Source: CAD feature listing. Evaluate the final solid. Frame: model axes, mm. A direction names the side the tool comes from. Give positions to 0.01 mm unless a question says otherwise; leave off trailing zeros. Order: outer loops, then holes, each group sorted by start corner. A loop starts at its lowest first (then second) coordinate and runs counter-clockwise, first axis right, second up. Notation, with made-up numbers: (11.5, 68) - (47.5, 68) arc R33 ccw to (47.5, 97) - close; hole circle Ø7 at (7, -25). An arc over 180 degrees is marked (long way). Use CSV: the item, a comma, the result in double quotes.
```python
from build123d import *

# Parameters (mm, degrees)
ESBO_O1_R                = 1.55
RESSALTO_EXTRUS_O1_DEPTH = 6
ESBO_O2_R                = 1.6
CORTE_EXTRUS_O1_DEPTH    = 10


with BuildPart() as part:
    # Esboço1 → Ressalto-extrusão1 (new body)
    with BuildSketch(Plane.XY):
        with BuildLine():
            Line((-117, -30), (-106, -30))
            ThreePointArc((-106, -30), (-80, -5.923190379), (-54, -30))
            Line((-54, -30), (0, -30))
            Line((0, -30), (54, -30))
            ThreePointArc((54, -30), (80, -5.923190379), (106, -30))
            Line((106, -30), (117, -30))
            Line((117, -30), (117, -14.523190379))
            Line((117, -14.523190379), (113, -14.523190379))
            Line((113, -14.523190379), (113, -15.923190379))
            Line((113, -15.923190379), (110, -15.923190379))
            Line((110, -15.923190379), (110, -14.523190379))
            Line((110, -14.523190379), (106, -14.523190379))
            Line((106, -14.523190379), (106, -11.323190379))
            Line((106, -11.323190379), (110, -11.323190379))
            Line((110, -11.323190379), (110, -9.923190379))
            Line((110, -9.923190379), (113, -9.923190379))
            Line((113, -9.923190379), (113, -11.323190379))
            Line((113, -11.323190379), (117, -11.323190379))
            Line((117, -11.323190379), (117, 4.076809621))
            Line((117, 4.076809621), (80, 4.076809621))
            ThreePointArc((80, 4.076809621), (62.485380172, -0.45995744), (49.375792338, -12.929234481))
            ThreePointArc((49.375792338, -12.929234481), (43.925093688, -18.113704991), (36.642872777, -20))
            Line((36.642872777, -20), (-36.642872777, -20))
            ThreePointArc((-36.642872777, -20), (-43.925093688, -18.113704991), (-49.375792338, -12.929234481))
            ThreePointArc((-49.375792338, -12.929234481), (-62.485380172, -0.45995744), (-80, 4.076809621))
            Line((-80, 4.076809621), (-117, 4.076809621))
            Line((-117, 4.076809621), (-117, -11.323190379))
            Line((-117, -11.323190379), (-113, -11.323190379))
            Line((-113, -11.323190379), (-113, -9.923190379))
            Line((-113, -9.923190379), (-110, -9.923190379))
            Line((-110, -9.923190379), (-110, -11.323190379))
            Line((-110, -11.323190379), (-106, -11.323190379))
            Line((-106, -11.323190379), (-106, -14.523190379))
            Line((-106, -14.523190379), (-110, -14.523190379))
            Line((-110, -14.523190379), (-110, -15.923190379))
            Line((-110, -15.923190379), (-113, -15.923190379))
            Line((-113, -15.923190379), (-113, -14.523190379))
            Line((-113, -14.523190379), (-117, -14.523190379))
            Line((-117, -14.523190379), (-117, -30))
        make_face()
        with Locations((-47.5, -22)):
            Circle(ESBO_O1_R, mode=Mode.SUBTRACT)
        with Locations((47.5, -22)):
            Circle(ESBO_O1_R, mode=Mode.SUBTRACT)
    extrude(amount=RESSALTO_EXTRUS_O1_DEPTH)

    # Esboço2 → Corte-extrusão1 (cut)
    with BuildSketch(Plane.XY.offset(6)):
        with Locations((-111, -1.923190379)):
            Circle(ESBO_O2_R)
        with Locations((111, -1.923190379)):
            Circle(ESBO_O2_R)
        with BuildLine():
            Line((-109.4, -19.923190379), (-109.4, -23.923190379))
            ThreePointArc((-109.4, -23.923190379), (-111, -25.523190379), (-112.6, -23.923190379))
            Line((-112.6, -23.923190379), (-112.6, -19.923190379))
            ThreePointArc((-112.6, -19.923190379), (-111, -18.323190379), (-109.4, -19.923190379))
        make_face()
        with BuildLine():
            Line((109.4, -19.923190379), (109.4, -23.923190379))
            ThreePointArc((109.4, -23.923190379), (111, -25.523190379), (112.6, -23.923190379))
            Line((112.6, -23.923190379), (112.6, -19.923190379))
            ThreePointArc((112.6, -19.923190379), (111, -18.323190379), (109.4, -19.923190379))
        make_face()
    extrude(amount=-CORTE_EXTRUS_O1_DEPTH, mode=Mode.SUBTRACT)


solid = part.part
```
Item 1: Section C-C on x = -73. Return the cut outline in (y, z), then the cut area to 3 significant figures.
Filled in:
outline,"(-6.88, 0) - (3.39, 0) - (3.39, 6) - (-6.88, 6) - close"
area,"61.6 mm2"
Item 2: First-contact query: pin 1 (3 mm diameter, centred on x = 23, z = 5, fed in from +Y). Flat tip, straight axial feed; report the tip coordinate or a pass-through.
Filled in:
pin 1,"stops at y = -20"
Item 3: Material intervals for line 1 (Y direction, x = 111, z = 2.95); line 2 (X direction, y = -13.5, z = 3); line 3 (X direction, y = -8.5, z = 0.65), sorted ascending. Write a range as from..to.
Filled in:
line 1,"y = -30..-25.52, -18.32..-15.92, -9.92..-3.52, -0.32..4.08"
line 2,"x = -106..-98.38, -61.62..-49, 49..61.62, 98.38..106"
line 3,"x = -117..-91.3, -68.7..-52.63, 52.63..68.7, 91.3..117"
Item 4: Set-up query: faces 1 (the flat face through (-108, -11.323, 3)), 2 (the cylindrical face through (62.71, -0.336, 2.958)), 3 (the flat face through (108, -14.523, 3)). Return all of +Z, -Z, +X, -X, +Y, -Y with unobstructed straight access to the full face (end or side cutting, diameter ignored); none if empty.
Filled in:
face 1,"+Z, -Z, -X"
face 2,"+Z, -Z, +Y"
face 3,"+Z, -Z, +X"
Item 5: Section B-B on z = 2. Count the separate pieces of the cut face and the enclosed holes in it, then the cut area to 3 significant figures.
Filled in:
separate pieces,"1"
enclosed holes,"6"
area,"3,260 mm2"
Item 6: Section A-A on x = 64. Return the cut outline in (y, z).
Filled in:
outline,"(-11.41, 0) - (0.33, 0) - (0.33, 6) - (-11.41, 6) - close"
Item 7: Mould query, pull axis X, two halves, no side actions, for faces 4 (the flat face through (108, -11.323, 3)), 5 (the flat face through (117, -4, 3)), 6 (the flat face through (-109.4, -22, 3)). Classes: released by +X, released by -X, zero draft, split by the parting line, or undercut.
Filled in:
face 4,"zero draft"
face 5,"released by +X"
face 6,"undercut"
